For this review, take the finished solid that the model builds, in its own axes (mm). A direction names the side the tool comes from. Give positions to 0.01 mm unless a question says otherwise; leave off trailing zeros. Write each loop counter-clockwise with the first axis right and the second up, starting at its lowest first coordinate (ties: lowest second). Pieces come first, ordered by that corner, then holes. Notation, with made-up numbers: (37.5, -6.5) -> (67.5, -6.5) arc R10 ccw to (67.5, -2.5) -> close; hole circle Ø9 at (83.5, -34). An arc over 180 degrees is marked (long way). Write item = value, one per line.
```python
from build123d import *

# Parameters (mm, degrees)
CYLINDER_R     = 6.1
CYLINDER_DEPTH = 15
BOX007_W       = 11.7
BOX007_H       = 15
BOX007_DEPTH   = 15
BOX_W          = 18
BOX_H          = 20
BOX_DEPTH      = 31
BOX002_W       = 43
BOX002_H       = 10
BOX002_DEPTH   = 35
FILLET_R       = 5
FILLET001_R    = 1
FILLET002_R    = 0.5


with BuildPart() as cylinder:
    # Cylinder → Cylinder (new body)
    with BuildSketch(Plane(origin=(10, 12, 8), x_dir=(1, 0, 0), z_dir=(0, -1, 0))):
        Circle(CYLINDER_R)
    extrude(amount=CYLINDER_DEPTH)


with BuildPart() as cube007:
    # Box007 → Box007 (new body)
    with BuildSketch(Plane(origin=(4.2, -3, -7), x_dir=(1, 0, 0), z_dir=(0, 0, 1))):
        with Locations((5.85, 7.5)):
            Rectangle(BOX007_W, BOX007_H)
    extrude(amount=BOX007_DEPTH)


with BuildPart() as cube:
    # Box → Box (new body)
    with BuildSketch(Plane(origin=(20, 0, 0), x_dir=(1, 0, 0), z_dir=(0, 0, 1))):
        with Locations((9, 10)):
            Rectangle(BOX_W, BOX_H)
    extrude(amount=BOX_DEPTH)


with BuildPart() as fillet002:
    # Box002 → Box002 (new body)
    with BuildSketch(Plane.XY):
        with Locations((21.5, 5)):
            Rectangle(BOX002_W, BOX002_H)
    extrude(amount=BOX002_DEPTH)

    # Cut: cut Cube
    add(cube.part, mode=Mode.SUBTRACT)

    # Cut001: cut Cube007
    add(cube007.part, mode=Mode.SUBTRACT)

    # Cut002: cut Cylinder
    add(cylinder.part, mode=Mode.SUBTRACT)

    # Fillet
    fillet_edges = [fillet002.edges().sort_by_distance(p)[0] for p in [
        (0, 5, 35),
        (43, 5, 35),
    ]]
    fillet(fillet_edges, radius=FILLET_R)

    # Fillet001
    fillet001_edges = [fillet002.edges().sort_by_distance(p)[0] for p in [
        (0, 5, 0),
        (4.2, 5, 0),
        (43, 5, 0),
        (38, 5, 0),
        (20, 5, 31),
        (20, 5, 0),
        (15.9, 5, 0),
    ]]
    fillet(fillet001_edges, radius=FILLET001_R)

    # Fillet002
    fillet002_edges = [fillet002.edges().sort_by_distance(p)[0] for p in [
        (38, 5, 31),
    ]]
    fillet(fillet002_edges, radius=FILLET002_R)


solid = fillet002.part
```
(1) For pin 1 (10 mm diameter, centred on x = 10, z = 8, fed in from -Y); pin 2 (3 mm diameter, centred on x = 9.5, y = 2, fed in from -Z); pin 3 (1.5 mm diameter, centred on x = 10, y = 1.5, fed in from -Z); pin 4 (5 mm diameter, centred on x = 27, y = 6, fed in from -Z), all flat-tipped, find the tip position at first contact; note any pin that passes through.
Answers below:
pin_1 = through
pin_2 = 13.76
pin_3 = 14.05
pin_4 = 31
(2) Take a section at D-D (x = 10). Write out the cut boundary in (y, z), plus the area to 3 significant figures.
Answers below:
outline = (0, 14.1) -> (10, 14.1) -> (10, 35) -> (0, 35) -> close
area = 209 mm^2
(3) The part is to be moulded in two halves that separate along X. For faces 3 (the face through (10, 5.1, 14.1)), 4 (the face through (43, 5, 15)), 5 (the face through (2, 5, 0)), say which applies: released by +X, released by -X, zero draft, split by the parting line, or undercut.
Answers below:
face_3 = undercut
face_4 = released by +X
face_5 = zero draft
(4) Take a section at C-C (y = 2.25). Write out the cut boundary in (x, z).
Answers below:
outline = (0, 1) arc R1 ccw to (1, 0) -> (3.2, 0) arc R1 ccw to (4.2, 1) -> (4.2, 6.11) arc R6.1 cw (long way) to (15.9, 6.45) -> (15.9, 1) arc R1 ccw to (16.9, 0) -> (19, 0) arc R1 ccw to (20, 1) -> (20, 30) arc R1 cw to (21, 31) -> (37.5, 31) arc R0.5 cw to (38, 30.5) -> (38, 1) arc R1 ccw to (39, 0) -> (42, 0) arc R1 ccw to (43, 1) -> (43, 30) arc R5 ccw to (38, 35) -> (5, 35) arc R5 ccw to (0, 30) -> close
(5) To check wall thickness, follow probe 1 along X at (y, z) = (3.75, 8); probe 2 along X at (y, z) = (3, 2); probe 3 along X at (y, z) = (6.5, 20.5). State the ranges of each line that lie inside material, in increasing order.
Answers below:
probe_1 = 0 to 3.9, 16.1 to 20, 38 to 43
probe_2 = 0 to 4.2, 15.9 to 20, 38 to 43
probe_3 = 0 to 20, 38 to 43
(6) Take a section at B-B (z = 21.5). Write out the cut boundary in (x, y), plus the area to 3 significant figures.
Answers below:
outline = (0, 0) -> (20, 0) -> (20, 10) -> (0, 10) -> close; (38, 0) -> (43, 0) -> (43, 10) -> (38, 10) -> close
area = 250 mm^2
(7) Take a section at A-A (z = 8). Write out the cut boundary in (x, y), plus the area to 3 significant figures.
Answers below:
outline = (0, 0) -> (3.9, 0) -> (3.9, 10) -> (0, 10) -> close; (16.1, 0) -> (20, 0) -> (20, 10) -> (16.1, 10) -> close; (38, 0) -> (43, 0) -> (43, 10) -> (38, 10) -> close
area = 128 mm^2
(8) Tool access review of faces 1 (the face through (19.699, 5.07, 0.285)), 2 (the face through (42.715, 5.07, 0.301)): name each direction out of +Z, -Z, +X, -X, +Y, -Y from which nothing blocks a thin tool from reaching the whole face with its end or side.
Answers below:
face_1 = -Z, +Y, -Y
face_2 = -Z, +X, +Y, -Y
